from build123d import *

# Parameters (mm, degrees)
SKETCH_1_R               = 4.4
SKETCH_1_R_2             = 2.55
EXTRUDE_1_DEPTH          = 1.6
CUT_EXTRUDE_1_DEPTH      = 1
CUT_EXTRUDE_1_DEPTH_BACK = 2.6


with BuildPart() as part:
    # Эскиз1 → Бобышка-Вытянуть1 (new body)
    with BuildSketch(Plane(origin=(0, 0, 0), x_dir=(1, 0, 0), z_dir=(0, 1, 0))):
        Circle(SKETCH_1_R)
        Circle(SKETCH_1_R_2, mode=Mode.SUBTRACT)
    extrude(amount=EXTRUDE_1_DEPTH)

    # Эскиз2 → Вырез-Вытянуть1 (cut, two sides)
    with BuildSketch(Plane(origin=(0, 1.6, 0), x_dir=(1, 0, 0), z_dir=(0, 1, 0))) as cut_extrude_1_sk:
        with BuildLine():
            Line((0, -4.4), (-0.509482587, -2.498585098))
            ThreePointArc((-0.509482587, -2.498585098), (-0.256035153, -2.537113714), (0, -2.55))
            Line((0, -2.55), (0.488419817, -4.372807574))
            ThreePointArc((0.488419817, -4.372807574), (0.244588096, -4.393196634), (0, -4.4))
        make_face()
    extrude(amount=CUT_EXTRUDE_1_DEPTH, mode=Mode.SUBTRACT)
    extrude(cut_extrude_1_sk.sketch, amount=-CUT_EXTRUDE_1_DEPTH_BACK, mode=Mode.SUBTRACT)


solid = part.part
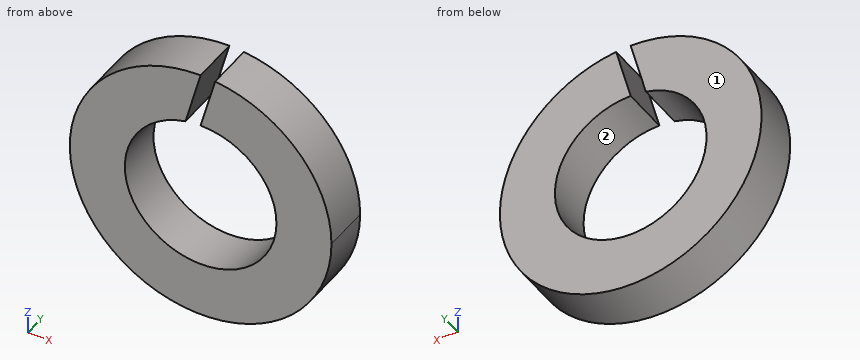
Check sheet for the modelled part. Datum: model origin and axes. Units: mm. Face numbers are marked on the shaded views. Give positions to 0.01 mm unless a question says otherwise; leave off trailing zeros. Write each loop counter-clockwise with the first axis right and the second up, starting at its lowest first coordinate (ties: lowest second). Pieces come first, ordered by that corner, then holes. Notation, with made-up numbers: (34, 63) -> (42, 63) arc R22 cw to (42, 90) -> close; hole circle Ø10 at (-25, -13). An arc over 180 degrees is marked (long way). Use one line per item in the form item = value. Start each with the question number.
1. Mould release check, pull along X, two halves, no side actions. Record for the marked faces 1 and 2: pulls with the +X half, pulls with the -X half, needs draft (parallel to the pull), parting line crosses it, or undercut.
2. Section check A-A (x = -1.25). Record the cut outline in (y, z).
3. Section check D-D (z = -3.5). Record the cut outline in (x, y).
4. Section check C-C (y = 0.95). Record the cut outline in (x, z), and give its area (3 significant figures).
5. Section check B-B (z = 3.75). Record the cut outline in (x, y).
6. Thickness scan on line 1 along X through (y, z) = (1.1, 0); line 2 along X through (y, z) = (1.1, 3.5); line 3 along Z through (x, y) = (-1, 0.4). Record the ranges inside material, lowest first. Write a range as from..to.
Conclusion:
q1.face_1 = needs draft
q1.face_2 = undercut
q2.outline = (0, -4.22) -> (1.6, -4.22) -> (1.6, -2.22) -> (0, -2.22) -> close; (0, 2.22) -> (1.6, 2.22) -> (1.6, 4.22) -> (0, 4.22) -> close
q3.outline = (-2.67, 0) -> (2.67, 0) -> (2.67, 1.6) -> (-2.67, 1.6) -> close
q4.outline = (-0.51, 2.5) -> (0, 4.4) arc R4.4 ccw (long way) to (0.49, 4.37) -> (0, 2.55) arc R2.55 cw (long way) to start
q4.area = 39.5 mm²
q5.outline = (-2.3, 0) -> (-0.17, 0) -> (-0.17, 1.6) -> (-2.3, 1.6) -> close; (0.32, 0) -> (2.3, 0) -> (2.3, 1.6) -> (0.32, 1.6) -> close
q6.line_1 = -4.4..-2.55, 2.55..4.4
q6.line_2 = -2.67..-0.24, 0.25..2.67
q6.line_3 = -4.28..-2.35, 2.35..4.28
